```python
from build123d import *

# Parameters (mm, degrees)
SKETCH_1_W                   = 50
SKETCH_1_H                   = 58
EXTRUDE_1_DEPTH              = 40
SKETCH_2_W                   = 32.792818714
SKETCH_2_H                   = 46
CUT_EXTRUDE_1_DEPTH          = 60
SKETCH_3_R                   = 7.5
CUT_EXTRUDE_2_DEPTH          = 35
HOLE_WIZARD_M5_1_D           = 5.5
HOLE_WIZARD_M5_1_DEPTH       = 17
HOLE_WIZARD_M5_1_CSINK_D     = 5.55
HOLE_WIZARD_M5_1_CSINK_ANGLE = 90
HOLE_WIZARD_M5_1_TIP         = 1.652366702
HOLE_WIZARD_M6_1_D           = 6.6
HOLE_WIZARD_M6_1_DEPTH       = 17
HOLE_WIZARD_M6_1_CSINK_D     = 6.65
HOLE_WIZARD_M6_1_CSINK_ANGLE = 90
HOLE_WIZARD_M6_1_TIP         = 1.982840043


with BuildPart() as part:
    # 草图1 → 凸台-拉伸1 (new body)
    with BuildSketch(Plane.XY):
        Rectangle(SKETCH_1_W, SKETCH_1_H)
    extrude(amount=EXTRUDE_1_DEPTH)

    # 草图2 → 切除-拉伸1 (cut)
    with BuildSketch(Plane.XY.offset(40)):
        with Locations((-21.396409357, 0)):
            Rectangle(SKETCH_2_W, SKETCH_2_H)
        with Locations((21.396409357, 0)):
            Rectangle(SKETCH_2_W, SKETCH_2_H)
    extrude(amount=-CUT_EXTRUDE_1_DEPTH, mode=Mode.SUBTRACT)

    # 草图3 → 切除-拉伸2 (cut)
    with BuildSketch(Plane.ZY.offset(5)):
        with Locations((20, 0)):
            Circle(SKETCH_3_R)
    extrude(amount=-CUT_EXTRUDE_2_DEPTH, mode=Mode.SUBTRACT)

    # M5 间隙槽口1
    with Locations(Plane(origin=(0, -29, 0), x_dir=(-1, 0, 0), z_dir=(0, -1, 0))):
        with Locations((-18, -4), (18, -4), (18, -36), (-18, -36)):
            CounterSinkHole(HOLE_WIZARD_M5_1_D / 2, HOLE_WIZARD_M5_1_CSINK_D / 2, depth=HOLE_WIZARD_M5_1_DEPTH, counter_sink_angle=HOLE_WIZARD_M5_1_CSINK_ANGLE)
            with Locations((0, 0, -(HOLE_WIZARD_M5_1_DEPTH + HOLE_WIZARD_M5_1_TIP / 2))):  # 118° drill point
                Cone(0, HOLE_WIZARD_M5_1_D / 2, HOLE_WIZARD_M5_1_TIP, mode=Mode.SUBTRACT)

    # M6 间隙槽口1
    with Locations(Plane(origin=(0, 29, 0), x_dir=(1, 0, 0), z_dir=(0, 1, 0))):
        with Locations((-15, -20), (15, -20)):
            CounterSinkHole(HOLE_WIZARD_M6_1_D / 2, HOLE_WIZARD_M6_1_CSINK_D / 2, depth=HOLE_WIZARD_M6_1_DEPTH, counter_sink_angle=HOLE_WIZARD_M6_1_CSINK_ANGLE)
            with Locations((0, 0, -(HOLE_WIZARD_M6_1_DEPTH + HOLE_WIZARD_M6_1_TIP / 2))):  # 118° drill point
                Cone(0, HOLE_WIZARD_M6_1_D / 2, HOLE_WIZARD_M6_1_TIP, mode=Mode.SUBTRACT)


solid = part.part
```
Geometry check sheet. Reference: the model listing, model coordinates, mm. A direction names the side the tool comes from. Coordinates: 2 decimals unless noted, no trailing zeros. Order: outer loops, then holes, each group sorted by start corner. A loop starts at its lowest first (then second) coordinate and runs counter-clockwise, first axis right, second up.
Item 1: Section check B-B (z = 20). Enter the section's corners in (x, y) (3 decimals), plus the area to 3 significant figures.
Item 2: Section check D-D (x = -8). Enter the section's corners in (y, z).
Item 3: Section check A-A (y = 0). Enter the section's corners in (x, z), plus the area to 3 significant figures.
Item 4: Tool access check on faces 1 (the cylindrical face through (17.619, 25.946, 22.008)), 2 (the cylindrical face through (17.642, -25.946, 33.273)), 3 (the flat face through (-5, 0, 29)), 4 (the flat face through (5, 0, 29)). Record the directions out of +Z, -Z, +X, -X, +Y, -Y that give a thin tool (end or side, any length) a straight path to the whole face; none if there is none.
Item 5: Section check C-C (y = -24.5). Enter the section's corners in (x, z), plus the area to 3 significant figures.
Item 6: Mould release check, pull along X, two halves, no side actions. Record for faces 5 (the cylindrical face through (-12.381, 25.946, 22.008)), 6 (the cylindrical face through (-0.07, 0.33, 12.507)), 7 (the flat face through (-25, 26, 20)): released by +X, released by -X, zero draft, split by the parting line, or undercut.
Item 7: Scan lines: line 1 along Z through (x, y) = (18, -26.4); line 2 along X through (y, z) = (-26.6, 36); line 3 along X through (y, z) = (27, 20). Record each from-to range of solid material in increasing order.
Item 8: Depth check by flat-ended pin: pin 1 (12 mm diameter, centred on y = 3.5, z = 32.5, fed in from +X); pin 2 (4 mm diameter, centred on y = 11, z = 21, fed in from -X); pin 3 (12 mm diameter, centred on y = 0, z = 20, fed in from +X); pin 4 (5.5 mm diameter, centred on x = -15, z = 20, fed in from +Y). Enter the tip coordinate at first touch or a pass-through.
Check sheet entries:
1. outline: (-25, -29) - (25, -29) - (25, -23) - (5, -23) - (5, -7.5) - (-5, -7.5) - (-5, -23) - (-25, -23) - close; (-25, 23) - (-18.3, 23) - (-18.3, 28.975) - (-18.325, 29) - (-25, 29) - close; (-11.7, 23) - (-5, 23) - (-5, 7.5) - (5, 7.5) - (5, 23) - (11.7, 23) - (11.7, 28.975) - (11.675, 29) - (-11.675, 29) - (-11.7, 28.975) - close; (18.3, 23) - (25, 23) - (25, 29) - (18.325, 29) - (18.3, 28.975) - close
1. area: 831 mm2
2. outline: (-29, 0) - (-23, 0) - (-23, 40) - (-29, 40) - close; (23, 0) - (29, 0) - (29, 40) - (23, 40) - close
3. outline: (-5, 0) - (5, 0) - (5, 12.5) - (-5, 12.5) - close; (-5, 27.5) - (5, 27.5) - (5, 40) - (-5, 40) - close
3. area: 250 mm2
4. face 1: +Y
4. face 2: -Y
4. face 3: +Z, -Z, -X
4. face 4: +Z, -Z, +X
5. outline: (-25, 0) - (25, 0) - (25, 40) - (-25, 40) - close; hole circle Ø5.5 at (-18, 4); hole circle Ø5.5 at (-18, 36); hole circle Ø5.5 at (18, 4); hole circle Ø5.5 at (18, 36)
5. area: 1,900 mm2
6. face 5: undercut
6. face 6: zero draft
6. face 7: released by -X
7. line 1: z = 0 to 1.25, 6.75 to 33.25, 38.75 to 40
7. line 2: x = -25 to -20.75, -15.25 to 15.25, 20.75 to 25
7. line 3: x = -25 to -18.3, -11.7 to 11.7, 18.3 to 25
8. pin 1: stops at x = 5
8. pin 2: stops at x = -5
8. pin 3: passes through
8. pin 4: stops at y = -23
